For this review, take the finished solid that the model builds, in its own axes (mm). A direction names the side the tool comes from. Give positions to 0.01 mm unless a question says otherwise; leave off trailing zeros. Loops run counter-clockwise (first coordinate to the right, second up) from the corner with the lowest first, then second, coordinate; pieces in that order, holes last. Notation, with made-up numbers: (72, 19) - (95, 19) arc R25 cw to (95, 35) - close; hole circle Ø3 at (63.25, 4). An arc over 180 degrees is marked (long way). Answer as CSV lines item,"result".
from build123d import *

# Parameters (mm, degrees)
F0_R     = 2.15265
F1_DEPTH = 6


with BuildPart() as f1:
    # F0 (on Top) → F1 (new body)
    with BuildSketch(Plane.XY):
        with BuildLine():
            ThreePointArc((-6.123496, -1.680862), (0, 6.35), (6.123496, -1.680862))
            Line((6.123496, -1.680862), (3.253002, -12.138271))
            ThreePointArc((3.253002, -12.138271), (5.400888, -23.200518), (15.499994, -28.199994))
            Line((15.499994, -28.199994), (116.995047, -28.199994))
            ThreePointArc((116.995047, -28.199994), (124.39015, -27.406244), (116.995047, -26.612494))
            Line((116.995047, -26.612494), (15.499994, -26.612494))
            ThreePointArc((15.499994, -26.612494), (6.663277, -22.237952), (4.783876, -12.558487))
            Line((4.783876, -12.558487), (7.65437, -2.101077))
            ThreePointArc((7.65437, -2.101077), (0, 7.9375), (-7.65437, -2.101077))
            Line((-7.65437, -2.101077), (-4.783876, -12.558487))
            ThreePointArc((-4.783876, -12.558487), (-6.663277, -22.237952), (-15.499994, -26.612494))
            Line((-15.499994, -26.612494), (-116.995047, -26.612494))
            ThreePointArc((-116.995047, -26.612494), (-124.39015, -27.406244), (-116.995047, -28.199994))
            Line((-116.995047, -28.199994), (-15.499994, -28.199994))
            ThreePointArc((-15.499994, -28.199994), (-5.400888, -23.200518), (-3.253002, -12.138271))
            Line((-3.253002, -12.138271), (-6.123496, -1.680862))
        make_face()
        with Locations((-120.65, -27.406244)):
            Circle(F0_R, mode=Mode.SUBTRACT)
        with Locations((120.65, -27.406244)):
            Circle(F0_R, mode=Mode.SUBTRACT)
    extrude(amount=F1_DEPTH)


solid = f1.part
1) Consider section B-B on y = -7. Write out the cut boundary in (x, z).
From the geometry:
outline,"(-6.31, 0) - (-4.66, 0) - (-4.66, 6) - (-6.31, 6) - close; (4.66, 0) - (6.31, 0) - (6.31, 6) - (4.66, 6) - close"
2) Machinability: for faces 1 (the flat face through (-66, -26.612, 3)), 2 (the flat face through (-67, -28.2, 3)), 3 (the flat face through (4.708, -6.836, 2.958)), which of the approach directions +Z, -Z, +X, -X, +Y, -Y give a long, thin tool a straight path to every point of the face, cutting with its end or side? Answer none if there is none.
From the geometry:
face 1,"+Z, -Z, +Y"
face 2,"+Z, -Z, -Y"
face 3,"+Z, -Z"
3) Consider section C-C on z = 4.65. Count the separate pieces of the cut face and the enclosed holes in it, and give its area (3 significant figures).
From the geometry:
separate pieces,"1"
enclosed holes,"2"
area,"526 mm^2"
4) Insertion check: P1, Ø2, axis at x = 76.5, z = 1, coming from the +Y side. The pin has a flat end and moves straight along its axis. Give the tip position at first contact, or say it passes through.
From the geometry:
P1,"stops at y = -26.61"
5) Wall thickness on line 1 (Y direction, x = 120.65, z = 2.8); line 2 (X direction, y = -28.5, z = 4.1); line 3 (Y direction, x = 53.5, z = 3.35): over which ranges is each line inside the solid? List them lowest first. Write a range as from..to.
From the geometry:
line 1,"y = -31.15..-29.56, -25.25..-23.67"
line 2,"x = -124.23..-122.5, -118.8..-117.07, 117.07..118.8, 122.5..124.23"
line 3,"y = -28.2..-26.61"
6) Consider section D-D on x = 0. Write out the cut boundary in (y, z).
From the geometry:
outline,"(6.35, 0) - (7.94, 0) - (7.94, 6) - (6.35, 6) - close"
7) Consider section A-A on x = 120.65. Write out the cut boundary in (y, z).
From the geometry:
outline,"(-31.15, 0) - (-29.56, 0) - (-29.56, 6) - (-31.15, 6) - close; (-25.25, 0) - (-23.67, 0) - (-23.67, 6) - (-25.25, 6) - close"
8) Draft analysis for pull direction Y (two halves, no side actions). For faces 4 (the flat face through (-6.24, -7.26, 2.96)), 5 (the flat face through (9, -26, 0)), 6 (the cylindrical face through (124.387, -27.56, 2.958)), state which applies: pulls with the +Y half, pulls with the -Y half, needs draft (parallel to the pull), parting line crosses it, or undercut.
From the geometry:
face 4,"undercut"
face 5,"needs draft"
face 6,"parting line crosses it"
